Could you check a few things on this drawing? It's one solid part, dimensions in mm from its lowest x, y, z. Round coordinates to 2 decimals unless told otherwise and drop trailing zeros. Write each loop counter-clockwise with the first axis right and the second up, starting at its lowest first coordinate (ties: lowest second). Pieces come first, ordered by that corner, then holes. Notation, with made-up numbers: (-34, 59.5) - (-15, 59.5) arc R15 ccw to (-15, 77.5) - close; hole circle Ø3 at (-24.5, 42.25). An arc over 180 degrees is marked (long way). Use one line per item in the form item = value. Start each with the question number.
1. I want a section at C-C, the plane y = 87.5. List the corners of the cut face in (x, z) for me.
2. I want a section at A-A, the plane y = 48.5. List the corners of the cut face in (x, z) for me (1 decimal), plus the area to 3 significant figures.
3. I want a section at B-B, the plane z = 3.5. State how many separate pieces and enclosed holes the cut face has, plus the area to 3 significant figures.
4. I want a section at D-D, the plane y = 119.5. List the corners of the cut face in (x, z) for me.
5. If I drill on line 1 along X through (y, z) = (57.5, 7) (1 decimal); line 2 along X through (y, z) = (61, 7.75) (1 decimal); line 3 along X through (y, z) = (104, 1.5) (1 decimal), over which ranges is the centre line in solid material (lowest first)?
6. Will this pin go through, and if not, where does the flat tip stop? pin 1 (4 mm diameter, centred on y = 66, z = 6.5, fed in from -X).
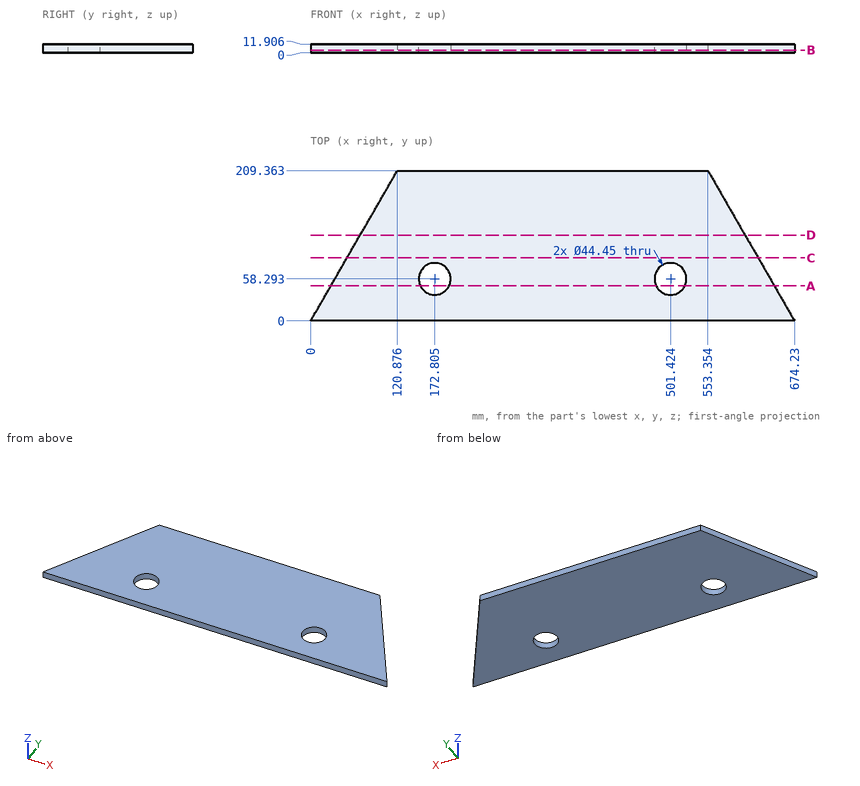
Model answer:
q1.outline = (50.52, 0) - (623.71, 0) - (623.71, 11.91) - (50.52, 11.91) - close
q2.outline = (28, 0) - (152.9, 0) - (152.9, 11.9) - (28, 11.9) - close; (192.8, 0) - (481.5, 0) - (481.5, 11.9) - (192.8, 11.9) - close; (521.4, 0) - (646.2, 0) - (646.2, 11.9) - (521.4, 11.9) - close
q2.area = 6,410 mm2
q3.separate_pieces = 1
q3.enclosed_holes = 2
q3.area = 113,000 mm2
q4.outline = (68.99, 0) - (605.24, 0) - (605.24, 11.91) - (68.99, 11.91) - close
q5.line_1 = 33.2 to 150.6, 195 to 479.2, 523.6 to 641
q5.line_2 = 35.2 to 150.7, 194.9 to 479.4, 523.5 to 639
q5.line_3 = 60 to 614.2
q6.pin_1 = 36.95
